Geometry: see drawing. Coordinates: mm, zero at the bounding-box minimum. A direction names the side the tool comes from. Coordinates: 2 decimals unless noted, no trailing zeros. Loops run counter-clockwise (first coordinate to the right, second up) from the corner with the lowest first, then second, coordinate; pieces in that order, holes last. Notation, with made-up numbers: (-20.5, 52) -> (3.5, 52) arc R25 cw to (3.5, 79) -> close; hole circle Ø11 at (-15.5, 67). An arc over 180 degrees is marked (long way). Put each result on its own line as item: value. Start each with the question number.
1) Contact query for flat-ended pins moving along their axis: P1, Ø2, axis at x = 148.5, z = 35, coming from the -Y side; P2, Ø1, axis at x = 95, z = 14.5, coming from the +Y side. Output: stop coordinate, or through.
2) Cut plane B-B (x = 182.5). Return the cut outline in (y, z).
3) Pull-direction query (X, two-part tool) for the marked faces 3, 4 and 5; classes: pulls with the +X half, pulls with the -X half, needs draft (parallel to the pull), parting line crosses it, or undercut.
4) Material intervals for L1, parallel to Y at x = 346, z = 38; L2, parallel to Y at x = 369, z = 5, sorted ascending.
5) Cut plane C-C (x = 365.5). Return the cut outline in (y, z).
6) Cut plane A-A (z = 8). Return the cut outline in (x, y).
7) Set-up query: the marked faces 1 and 2. Return all of +Z, -Z, +X, -X, +Y, -Y with unobstructed straight access to the full face (end or side cutting, diameter ignored); none if empty.
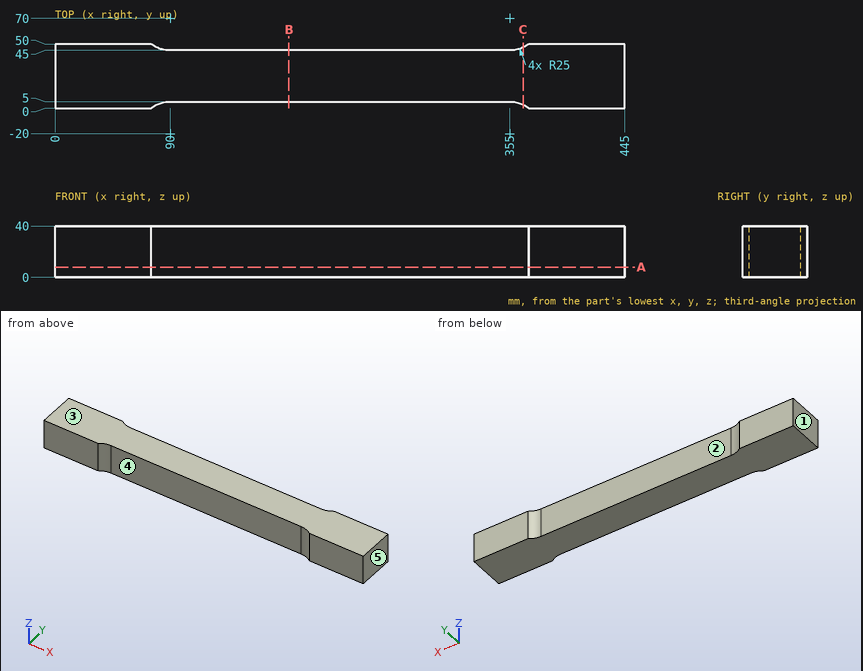
Results found:
1. P1: stops at y = 5
1. P2: stops at y = 45
2. outline: (5, 0) -> (45, 0) -> (45, 40) -> (5, 40) -> close
3. face 3: needs draft
3. face 4: undercut
3. face 5: pulls with the +X half
4. L1: y = 5 to 45
4. L2: y = 0.71 to 49.29
5. outline: (2.69, 0) -> (47.31, 0) -> (47.31, 40) -> (2.69, 40) -> close
6. outline: (0, 0) -> (75, 0) arc R25 cw to (90, 5) -> (355, 5) arc R25 cw to (370, 0) -> (445, 0) -> (445, 50) -> (370, 50) arc R25 cw to (355, 45) -> (90, 45) arc R25 cw to (75, 50) -> (0, 50) -> close
7. face 1: +Z, -Z, -X, +Y, -Y
7. face 2: +Z, -Z, +Y
